Check sheet for the modelled part. Datum: model origin and axes. Units: mm. A direction names the side the tool comes from. Give positions to 0.01 mm unless a question says otherwise; leave off trailing zeros. Order: outer loops, then holes, each group sorted by start corner. A loop starts at its lowest first (then second) coordinate and runs counter-clockwise, first axis right, second up. Notation, with made-up numbers: M -26,-21 L 1,-21 A20 ccw 1,-15 Z; hole C 73.25,84 d7. An arc over 180 degrees is marked long. Answer in a Markdown table with one row per item. Add a question column.
from build123d import *

# Parameters (mm, degrees)
F1_DEPTH         = 4.5
F3_DEPTH         = 1
F3_COPIES2_COUNT = 2
F5_DEPTH         = 3
F6_R             = 3.25
F7_DEPTH         = 3
F8_R             = 2
F9_DEPTH         = 20
F10_W            = 1
F10_H            = 6.5
F11_DEPTH        = 1.5
F12_R            = 1


# Not quite as in the source:
# - a pattern or mirror of a feature is missing from the dataset's text; its kind, count and spacing are read off the source's solid


with BuildPart() as f1:
    # F0 (on Front) → F1 (new body, symmetric)
    with BuildSketch(Plane.XZ):
        with BuildLine():
            Line((-8.5, 33.6271340575), (-8.5, 25.6271340575))
            ThreePointArc((-8.5, 25.6271340575), (0, -27), (8.5, 25.6271340575))
            Line((8.5, 25.6271340575), (8.5, 33.6271340575))
            Line((8.5, 33.6271340575), (7.5, 33.6271340575))
            Line((7.5, 33.6271340575), (7.5, 24.894778569))
            ThreePointArc((7.5, 24.894778569), (0, -26), (-7.5, 24.894778569))
            Line((-7.5, 24.894778569), (-7.5, 33.6271340575))
            Line((-7.5, 33.6271340575), (-8.5, 33.6271340575))
        make_face()
    extrude(amount=F1_DEPTH, both=True)

    # F2 (on face) → F3 (join)
    with BuildSketch(Plane.XZ.offset(4.5)):
        with BuildLine():
            Line((-8.5, 25.6271340575), (-8.5, 33.6271340575))
            Line((-8.5, 33.6271340575), (-16.5, 21.3717102732))
            ThreePointArc((-16.5, 21.3717102732), (-12.6797932907, 23.8374252407), (-8.5, 25.6271340575))
        make_face()
    f3 = extrude(amount=-F3_DEPTH)

    # F3_copies: F3 across plane
    add(f3.mirror(Plane.ZX))

    # F3_copies1: F3 across plane
    add(f3.mirror(Plane(origin=(0, 0, 0), x_dir=(0, 0, 1), z_dir=(1, 0, 0))))

    # F3_copies2: F3 ×2 about axis
    f3_copies2_axis = Axis((0, 0, 0), (0, 0, 1))
    for i in range(1, F3_COPIES2_COUNT):
        add(f3.rotate(f3_copies2_axis, i * 360 / F3_COPIES2_COUNT))

    # F4 (on face) → F5 (join)
    with BuildSketch(Plane(origin=(-8.5, 0, 0), x_dir=(0, -1, 0), z_dir=(-1, 0, 0))):
        Polygon((-3.25, 31.5035224323), (-3.25, 27.7507456826), (0, 25.8743573077), (3.25, 27.7507456826), (3.25, 31.5035224323), (0, 33.3799108072), align=None)
    extrude(amount=F5_DEPTH)

    # F6 (on face) → F7 (join)
    with BuildSketch(Plane.YZ.offset(8.5)):
        with Locations((0, 29.6271340575)):
            Circle(F6_R)
    extrude(amount=F7_DEPTH)

    # F8 (on face) → F9 (join)
    with BuildSketch(Plane(origin=(7.5, 0, 0), x_dir=(0, -1, 0), z_dir=(-1, 0, 0))):
        with Locations((0, 29.6271340575)):
            Circle(F8_R)
    extrude(amount=F9_DEPTH)

    # F10 (on face) → F11 (cut)
    with BuildSketch(Plane.YZ.offset(11.5)):
        with Locations((0, 29.6271340575)):
            Rectangle(F10_W, F10_H)
    extrude(amount=-F11_DEPTH, mode=Mode.SUBTRACT)

    # F12
    f12_edges = [f1.edges().sort_by_distance(p)[0] for p in [
        (11.5, -3.25, 29.627134),
        (11.5, 2.468552, 31.741076),
        (11.5, 2.468552, 27.513192),
    ]]
    fillet(f12_edges, radius=F12_R)


solid = f1.part
Q1. Cross-section at A-A (z = 6). Record the boundary of the cut face in (x, y), and give its area (3 significant figures).
Q2. Cross-section at C-C (z = 15). Record the boundary of the cut face in (x, y), and give its area (3 significant figures).
Q3. Cross-section at D-D (x = -6.5). Record the boundary of the cut face in (y, z), and give its area (3 significant figures).
Q4. Go/stop test with flat-tipped pins: pin 1 (1.1 mm diameter, centred on y = 0, z = 29.5, fed in from +X); pin 2 (4.5 mm diameter, centred on y = 0, z = 29.5, fed in from -X); pin 3 (3 mm diameter, centred on y = 1, z = -12, fed in from +X); pin 4 (4 mm diameter, centred on x = -1.5, z = 25.5, fed in from +Y). Record where each tip stops, or that it passes through.
Q5. Cross-section at B-B (x = -13.5). Record the boundary of the cut face in (y, z), and give its area (3 significant figures).
Q6. Draft check along Y on faces 4 (the cylindrical face through (9.486, 1.5, 26.744)), 5 (the cylindrical face through (0.11, 0.26, 31.61)), 6 (the flat face through (11, 3.5, 27)), 7 (the flat face through (-12.5, 0, 30)). Enter one of: pulls with the +Y half, pulls with the -Y half, needs draft (parallel to the pull), parting line crosses it, or undercut.
Q7. Thickness scan on probe 1 along X at (y, z) = (-1, 31.5); probe 2 along Z at (x, y) = (0, 0.25); probe 3 along X at (y, z) = (0.5, 0). Record the ranges inside material, lowest first.
Q8. Tool access check on faces 1 (the flat face through (-12.44, -4.01, 27.59)), 2 (the flat face through (-10, 3.25, 30)), 3 (the flat face through (11.5, -1, 30)). Record the directions out of +Z, -Z, +X, -X, +Y, -Y that give a thin tool (end or side, any length) a straight path to the whole face; none if there is none.
Values follow:
| question | item | result |
|---|---|---|
| 1 | outline | M -26.32,-4.5 L -25.3,-4.5 L -25.3,4.5 L -26.32,4.5 Z; M 25.3,-4.5 L 26.32,-4.5 L 26.32,4.5 L 25.3,4.5 Z |
| 1 | area | 18.5 mm² |
| 2 | outline | M -22.45,-4.5 L -21.24,-4.5 L -21.24,4.5 L -22.45,4.5 Z; M 21.24,-4.5 L 22.45,-4.5 L 22.45,4.5 L 21.24,4.5 Z |
| 2 | area | 21.8 mm² |
| 3 | outline | M -4.5,-26.21 L 4.5,-26.21 L 4.5,-25.17 L -4.5,-25.17 Z; C 0,29.63 d4 |
| 3 | area | 21.9 mm² |
| 4 | pin 1 | x = 11.5 |
| 4 | pin 2 | x = -12.5 |
| 4 | pin 3 | x = 24.87 |
| 4 | pin 4 | through |
| 5 | outline | M -4.5,-23.38 L 4.5,-23.38 L 4.5,-22.22 L -4.5,-22.22 Z; M -4.5,22.22 L 4.5,22.22 L 4.5,25.97 L 3.5,25.97 L 3.5,23.38 L -3.5,23.38 L -3.5,25.97 L -4.5,25.97 Z |
| 5 | area | 26.1 mm² |
| 6 | face 4 | undercut |
| 6 | face 5 | parting line crosses it |
| 6 | face 6 | undercut |
| 6 | face 7 | needs draft |
| 7 | probe 1 | -11.5 to -7.5, 7.5 to 11.5 |
| 7 | probe 2 | -27 to -26, 27.64 to 31.61 |
| 7 | probe 3 | -27 to -26, 26 to 27 |
| 8 | face 1 | +Z, -X, -Y |
| 8 | face 2 | +Z, -X |
| 8 | face 3 | +Z, +X |
